Design review of the part built by this model. Coordinates are the model's own, in mm. A direction names the side the tool comes from. Coordinates: 2 decimals unless noted, no trailing zeros. Answer in a Markdown table with one row per item. Add a question column.
Item 1: Draft analysis for pull direction X (two halves, no side actions). For faces 1 (the face through (-11, 3.175, -17)), 2 (the face through (-1.838, 2, -2)), state which applies: released by +X, released by -X, zero draft, split by the parting line, or undercut.
Item 2: To check wall thickness, follow line 1 (X direction, y = 1.8, z = -70); line 2 (X direction, y = 0.35, z = -68); line 3 (Z direction, x = 11, y = 1.05). State the ranges of each line that lie inside material, in increasing order.
Item 3: For faces 3 (the face through (1.662, 2, -2)), 4 (the face through (-72, 2, -80)), list the 3-axis set-ups (+Z, -Z, +X, -X, +Y, -Y) from which the entire face can be reached by the end or side of a thin tool; tool diameter is ignored.
Item 4: Clearance check with flat-ended pins moving along their axes: P1, Ø1.6, axis at y = 1, z = -3, coming from the -X side; P2, Ø10, axis at x = 12, z = -19.5, coming from the +Y side (3 decimals). State where each tip first meets the part, or that it passes through.
from build123d import *

# Parameters (mm, degrees)
BOSS_EXTRUDE2_DEPTH = 3.175
SKETCH2_W           = 3.5
SKETCH2_H           = 5
CUT_EXTRUDE1_DEPTH  = 114.181630536


with BuildPart() as part:
    # Sketch1 → Boss-Extrude2 (new body)
    with BuildSketch(Plane(origin=(0, 0, 0), x_dir=(1, 0, 0), z_dir=(0, 1, 0))):
        with BuildLine():
            add(Edge.make_bspline(
                [(-63.153287392, 80.000005207), (-62.690087061, 79.114787151), (-61.425361806, 76.720578148), (-59.365002639, 72.921941484), (-56.178071622, 67.245371862), (-52.217635229, 60.563206955), (-47.510051679, 53.209135647), (-42.857631564, 46.523268117), (-36.745022116, 38.503236865), (-29.311161013, 30.160913336), (-20.883951302, 22.824255391), (-13.153033777, 18.042065099), (-6.254689992, 15.505931404), (0, 14.747034298), (6.254689993, 15.505931404), (13.153033778, 18.042065099), (20.883951303, 22.824255391), (29.311161014, 30.160913336), (36.745022116, 38.503236864), (42.857631564, 46.523268116), (47.510051679, 53.209135647), (52.217635229, 60.563206955), (56.178071622, 67.245371862), (59.365002639, 72.921941484), (61.425361806, 76.720578148), (62.690087062, 79.114787152), (63.153287392, 80.000005207)],
                knots=[0.075765822, 0.075765822, 0.075765822, 0.075765822, 0.083776621, 0.097650734, 0.111524847, 0.139273072, 0.167021297, 0.194769522, 0.222517748, 0.278014198, 0.333510649, 0.389007099, 0.44450355, 0.5, 0.55549645, 0.610992901, 0.666489351, 0.721985802, 0.777482252, 0.805230478, 0.832978703, 0.860726928, 0.888475153, 0.902349266, 0.916223379, 0.924234178, 0.924234178, 0.924234178, 0.924234178], degree=3))
            Line((63.153287392, 80.000005207), (80, 80))
            add(Edge.make_bspline(
                [(-80, 80), (0, -80), (80, 80)],
                knots=[0.056028396, 0.056028396, 0.056028396, 0.943971604, 0.943971604, 0.943971604], degree=2))
            Line((-80, 80), (-63.153287392, 80.000005207))
        make_face()
    extrude(amount=BOSS_EXTRUDE2_DEPTH)

    # Sketch2 → Cut-Extrude1 (cut, through all)
    with BuildSketch(Plane(origin=(0, 3.175, 0), x_dir=(1, 0, 0), z_dir=(0, 1, 0))):
        with Locations((-0.08811954, 2.5)):
            Rectangle(SKETCH2_W, SKETCH2_H)
    extrude(amount=-CUT_EXTRUDE1_DEPTH, mode=Mode.SUBTRACT)


solid = part.part
Answers:
| question | item | result |
|---|---|---|
| 1 | face 1 | zero draft |
| 1 | face 2 | undercut |
| 2 | line 1 | x = -74.83 to -57.72, 57.72 to 74.83 |
| 2 | line 2 | x = -73.76 to -56.58, 56.58 to 73.76 |
| 2 | line 3 | z = -17.36 to -1.51 |
| 3 | face 3 | +Z, +Y, -Y |
| 3 | face 4 | -Z, +X, -X, +Y, -Y |
| 4 | P1 | stops at x = -17.44 |
| 4 | P2 | stops at y = 3.175 |
